```python
from build123d import *

# Parameters (mm, degrees)
F1_DEPTH = 40
F0_W     = 120
F0_H     = 160
F0_R     = 5
F2_DEPTH = 10
F3_R     = 10


with BuildPart() as f1:
    # F0 (on Top) → F1 (new body)
    with BuildSketch(Plane.XY):
        Polygon((16.638367, -41.511019), (43.191836, -11.595918), (-16.638367, 41.511019), (-43.191836, 11.595918), align=None)
    extrude(amount=F1_DEPTH)

    # F0 (on Top) → F2 (join)
    with BuildSketch(Plane.XY):
        Rectangle(F0_W, F0_H)
        with Locations((-50, -70)):
            Circle(F0_R, mode=Mode.SUBTRACT)
        with Locations((50, -70)):
            Circle(F0_R, mode=Mode.SUBTRACT)
        Polygon((-16.638367, 41.511019), (43.191836, -11.595918), (16.638367, -41.511019), (-43.191836, 11.595918), align=None, mode=Mode.SUBTRACT)
        with Locations((-50, 70)):
            Circle(F0_R, mode=Mode.SUBTRACT)
        with Locations((50, 70)):
            Circle(F0_R, mode=Mode.SUBTRACT)
    extrude(amount=F2_DEPTH)

    # F3
    f3_edges = [f1.edges().sort_by_distance(p)[0] for p in [
        (13.276734, 14.957551, 40),
        (-13.276734, -14.957551, 40),
    ]]
    fillet(f3_edges, radius=F3_R)


solid = f1.part
```
Can you work these out from the model? Positions are in its coordinate system, mm. A direction names the side the tool comes from. Give positions to 0.01 mm unless a question says otherwise; leave off trailing zeros. Write each loop counter-clockwise with the first axis right and the second up, starting at its lowest first coordinate (ties: lowest second). Pieces come first, ordered by that corner, then holes. Notation, with made-up numbers: (0.5, 13) -> (50.5, 13) arc R31 ccw to (50.5, 39) -> close; hole circle Ø7 at (66, 16.5). An arc over 180 degrees is marked (long way). One line per item, written item: value.
Q1. Imagine slicing it at B-B on x = 50. Please give me the cut outline in (y, z).
Results found:
outline: (-80, 0) -> (-75, 0) -> (-75, 10) -> (-80, 10) -> close; (-65, 0) -> (65, 0) -> (65, 10) -> (-65, 10) -> close; (75, 0) -> (80, 0) -> (80, 10) -> (75, 10) -> close
Q2. We'd pull the mould along X, two halves only. Please class faces 1 (the face through (60, -1, 5)), 2 (the face through (-1, -80, 5)), 3 (the face through (-54, -67, 5)): +X half, -X half, draft (parallel to the pull), parting line (faces both ways), or undercut.
Results found:
face 1: +X half
face 2: draft
face 3: undercut
Q3. Which directions (+Z, -Z, +X, -X, +Y, -Y) give clear straight access to the entire face, cutting with the end or side of a thin tool? Please do faces 4 (the face through (-13.696, -14.586, 19.86)), 5 (the face through (29.73, -26.76, 24.79)), 6 (the face through (-29.73, 26.76, 24.79)), 7 (the face through (13.696, 14.586, 19.86)), 8 (the face through (12, 19, 10)).
Results found:
face 4: +Z, -X, -Y
face 5: +Z, +X, -Y
face 6: +Z, -X, +Y
face 7: +Z, +X, +Y
face 8: +Z
Q4. Please list where these lines run through material, in increasing order: line 1 (Y direction, x = -50, z = 3.25); line 2 (Z direction, x = -23, y = -60.5); line 3 (Y direction, x = -14, z = 16.5). Write a range as [from, to].
Results found:
line 1: y = [-80, -75], [-65, 65], [75, 80]
line 2: z = [0, 10]
line 3: y = [-14.32, 39.17]
Q5. For P1, Ø1, axis at x = -42.5, z = 27.5, coming from the +Y side; P2, Ø12, axis at x = 13.5, z = 28, coming from the +Y side; P3, Ø13, axis at x = -50, y = -70, coming from the +Z side, each with a flat end and sliding along its axis, tell me the tip position at first contact or that it passes through.
Results found:
P1: stops at y = 12.94
P2: stops at y = 20.09
P3: stops at z = 10
Q6. Imagine slicing it at C-C on z = 26.5. Please give me the cut outline in (x, y), and give its area (3 significant figures).
Results found:
outline: (-43.19, 11.6) -> (16.64, -41.51) -> (43.19, -11.6) -> (-16.64, 41.51) -> close
area: 3,200 mm^2
Q7. Imagine slicing it at A-A on y = 70. Please give me the cut outline in (x, z).
Results found:
outline: (-60, 0) -> (-55, 0) -> (-55, 10) -> (-60, 10) -> close; (-45, 0) -> (45, 0) -> (45, 10) -> (-45, 10) -> close; (55, 0) -> (60, 0) -> (60, 10) -> (55, 10) -> close
